from build123d import *

# Parameters (mm, degrees)
SKETCH1_R           = 10
BOSS_EXTRUDE1_DEPTH = 145
SKETCH2_R           = 10
SKETCH2_R_2         = 7
CUT_EXTRUDE1_DEPTH  = 97
FILLET1_R           = 1
CUT_LOFT1_START     = -2.5
CUT_LOFT1_DEPTH     = 5


# Read off the part's stored shape, not the designer's step: Cut-Loft1
with BuildPart() as part:
    # Sketch1 → Boss-Extrude1 (new body)
    with BuildSketch(Plane(origin=(0, 0, 0), x_dir=(0, 0, -1), z_dir=(1, 0, 0))):
        Circle(SKETCH1_R)
    extrude(amount=-BOSS_EXTRUDE1_DEPTH)

    # Sketch2 → Cut-Extrude1 (cut)
    with BuildSketch(Plane(origin=(-60, 0, 0), x_dir=(0, 0, -1), z_dir=(1, 0, 0))):
        Circle(SKETCH2_R)
        Circle(SKETCH2_R_2, mode=Mode.SUBTRACT)
    extrude(amount=-CUT_EXTRUDE1_DEPTH, mode=Mode.SUBTRACT)

    # Fillet1
    fillet1_edges = [part.edges().sort_by_distance(p)[0] for p in [
        (-60, 0, 7),
    ]]
    fillet(fillet1_edges, radius=FILLET1_R)

    # Cut-Loft1 outline → Cut-Loft1 (cut)
    with BuildSketch(Plane(origin=(0, 0, 0), x_dir=(1, 0, 0), z_dir=(0, 1, 0)).offset(CUT_LOFT1_START)):
        Polygon((-65, -8), (-65, -6.008348415), (-145, -4.508348415), (-145, -8), align=None)
    extrude(amount=CUT_LOFT1_DEPTH, mode=Mode.SUBTRACT)


solid = part.part
Verification items for the finished model (mm, model axes). Round coordinates to 2 decimals unless told otherwise and drop trailing zeros. Loops run counter-clockwise (first coordinate to the right, second up) from the corner with the lowest first, then second, coordinate; pieces in that order, holes last. Notation, with made-up numbers: (46, 46) - (51, 46) arc R28 ccw to (51, 69) - close; hole circle Ø11 at (74, 41.25). An arc over 180 degrees is marked (long way). Answer in a Markdown table with one row per item. Add a question column.
Q1. Section check C-C on x = -24. Enter the section's corners in (y, z).
Q2. Material ranges on line 1 (Y direction, x = -114.5, z = 5.75); line 2 (X direction, y = 8.75, z = 0); line 3 (Z direction, x = -94.5, y = 5.25), recorded low to high.
Q3. Gauge pin test, flat ends, axial feed: pin 1 (8 mm diameter, centred on x = -47, y = -5.5, fed in from -Z); pin 2 (10 mm diameter, centred on x = -110, z = -8, fed in from -Y); pin 3 (0.8 mm diameter, centred on y = 0.5, z = 6.5, fed in from -X). Record the tip position at first contact, or that the pin passes through.
Q4. Section check D-D on x = -96. Enter the section's corners in (y, z), plus the area to 3 significant figures.
Q5. Release check for a two-part mould opening along Y. For faces 1 (the face through (-102.412, -2.681, -6.466)), 2 (the face through (-60, 8.2, 0)) record: pulls with the +Y half, pulls with the -Y half, needs draft (parallel to the pull), parting line crosses it, or undercut.
Q6. Section check B-B on y = 0. Enter the section's corners in (x, z).
Q7. Section check A-A on z = 0. Enter the section's corners in (x, y), plus the area to 3 significant figures.
Found:
| question | item | result |
|---|---|---|
| 1 | outline | circle Ø20 at (0, 0) |
| 2 | line 1 | y = -3.99 to -2.5, 2.5 to 3.99 |
| 2 | line 2 | x = -60 to 0 |
| 2 | line 3 | z = -4.63 to 4.63 |
| 3 | pin 1 | stops at z = -9.89 |
| 3 | pin 2 | stops at y = -6.32 |
| 3 | pin 3 | stops at x = -65 |
| 4 | outline | (-2.5, 5.43) - (-2.5, 6.54) arc R7 ccw (long way) to (2.5, 6.54) - (2.5, 5.43) - close |
| 4 | area | 147 mm² |
| 5 | face 1 | parting line crosses it |
| 5 | face 2 | needs draft |
| 6 | outline | (-145, -7) - (-61, -7) arc R1 cw to (-60, -8) - (-60, -10) - (0, -10) - (0, 10) - (-60, 10) - (-60, 8) arc R1 cw to (-61, 7) - (-65, 7) - (-65, 6.01) - (-145, 4.51) - close |
| 7 | outline | (-145, -7) - (-61, -7) arc R1 cw to (-60, -8) - (-60, -10) - (0, -10) - (0, 10) - (-60, 10) - (-60, 8) arc R1 cw to (-61, 7) - (-145, 7) - close |
| 7 | area | 2,390 mm² |
